Can you work these out from the model? Positions are in its coordinate system, mm. Face numbers are marked on the shaded views. A direction names the side the tool comes from. Round coordinates to 2 decimals unless told otherwise and drop trailing zeros. Loops run counter-clockwise (first coordinate to the right, second up) from the corner with the lowest first, then second, coordinate; pieces in that order, holes last. Notation, with made-up numbers: M 22,-27.5 L 59,-27.5 A20 cw 59,-20.5 Z; hole C 24,-3 d11. An arc over 180 degrees is marked long. Answer as CSV lines item,"result".
from build123d import *

# Parameters (mm, degrees)
SKETCH_W        = 16.6
SKETCH_H        = 25
PAD_DEPTH       = 2
SKETCH001_W     = 19.4
SKETCH001_H     = 30
PAD001_DEPTH    = 6
POCKET_DEPTH    = 30.001
SKETCH003_W     = 15.087606
SKETCH003_H     = 23.432943
POCKET001_DEPTH = 3
POCKET002_DEPTH = 23


with BuildPart() as part:
    # Sketch → Pad (new body)
    with BuildSketch(Plane.XY):
        with Locations((0, -0.5)):
            Rectangle(SKETCH_W, SKETCH_H)
    extrude(amount=PAD_DEPTH)

    # Sketch001 (on Face5 of Pad) → Pad001 (join)
    with BuildSketch(Plane(origin=(0, 0, 0), x_dir=(1, 0, 0), z_dir=(0, 0, -1))):
        with Locations((0, -1)):
            Rectangle(SKETCH001_W, SKETCH001_H)
    extrude(amount=PAD001_DEPTH)

    # Sketch002 (on Face1 of Pad001) → Pocket (cut, through all)
    with BuildSketch(Plane.XZ.offset(14)):
        with BuildLine():
            ThreePointArc((-9.5, 0), (-8.500128, -3.558582), (-5.793155, -6.075635))
            Line((10.964428, -0.352326), (-5.793155, -6.075635))
            Line((10.964428, -0.352326), (10.392425, -13.720259))
            Line((10.392425, -13.720259), (-15.284175, -12.512696))
            Line((-9.5, 2.985816), (-15.284175, -12.512696))
            Line((-9.5, 0), (-9.5, 2.985816))
        make_face()
    extrude(amount=-POCKET_DEPTH, mode=Mode.SUBTRACT)

    # Sketch003 (on Face12 of Pocket) → Pocket001 (cut)
    with BuildSketch(Plane.XY.offset(2)):
        with Locations((0.03044, -0.598662)):
            Rectangle(SKETCH003_W, SKETCH003_H)
    extrude(amount=-POCKET001_DEPTH, mode=Mode.SUBTRACT)

    # Sketch004 (on Face13 of Pocket001) → Pocket002 (cut)
    with BuildSketch(Plane.XZ.offset(-11.117809)):
        with BuildLine():
            Line((7.061974, 0.986589), (-7.423936, 0))
            ThreePointArc((-7.423936, 0), (-5.193689, -5.663316), (-0.979385, -10.054988))
            Line((-0.979385, -10.054988), (7.061974, 0.986589))
        make_face()
    extrude(amount=POCKET002_DEPTH, mode=Mode.SUBTRACT)


solid = part.part
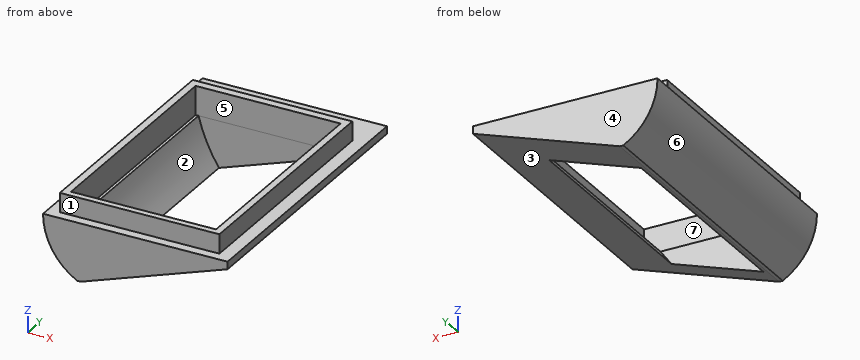
Item 1: If we section it at A-A on z = 0.5: Write out the boundary of the cut face in (x, y).
Output:
outline,"M -8.3,-13 L 8.3,-13 L 8.3,12 L -8.3,12 Z; hole M -7.51,-12.32 L 7.57,-12.32 L 7.57,11.12 L -7.51,11.12 Z"
Item 2: If we section it at B-B on x = -0.5: Write out the boundary of the cut face in (y, z), then the cut area to 3 significant figures.
Output:
outline,"M -14,-4.27 L -11.88,-4.27 L -11.88,-1 L -12.32,-1 L -12.32,2 L -13,2 L -13,0 L -14,0 Z; M 11.12,-4.27 L 16,-4.27 L 16,0 L 12,0 L 12,2 L 11.12,2 Z"
area,"32.6 mm2"
Item 3: We'd pull the mould along Y, two halves only. Please class the marked faces 4, 5, 6 and 7: released by +Y, released by -Y, zero draft, split by the parting line, or undercut.
Output:
face 4,"released by +Y"
face 5,"undercut"
face 6,"zero draft"
face 7,"undercut"
Item 4: On a 3-axis mill with a long thin cutter (end or side, diameter ignored), from which of +Z, -Z, +X, -X, +Y, -Y can I reach the whole of each face in a straight line? I mean the marked faces 1, 2 and 3. Say none if no direction works.
Output:
face 1,"+Z, +X, -X, -Y"
face 2,"+Z"
face 3,"-Z, +X, +Y, -Y"
Item 5: Will these pins go through, and if not, where does the flat tip stop? pin 1 (1.6 mm diameter, centred on x = -0.5, z = 1.5, fed in from +Y); pin 2 (1.6 mm diameter, centred on x = -2, z = 1, fed in from -Y); pin 3 (1.5 mm diameter, centred on y = 9.5, z = 1, fed in from -X).
Output:
pin 1,"stops at y = 12"
pin 2,"stops at y = -13"
pin 3,"stops at x = -8.3"
Item 6: If I drill on line 1 along Y through (x, z) = (2, 1); line 2 along Y through (x, z) = (0.5, -0.5); line 3 along X through (y, z) = (7.5, 0.75), over which ranges is the centre line in solid material (lowest first)? Write a range as from..to.
Output:
line 1,"y = -13..-12.32, 11.12..12"
line 2,"y = -14..-12.32, 11.12..16"
line 3,"x = -8.3..-7.51, 7.57..8.3"
